Can you work these out from the drawing? Everything is in mm from the part's minimum corner. A direction names the side the tool comes from. Round coordinates to 2 decimals unless told otherwise and drop trailing zeros. Order: outer loops, then holes, each group sorted by start corner. A loop starts at its lowest first (then second) coordinate and runs counter-clockwise, first axis right, second up. Notation, with made-up numbers: M 61.5,-31 L 108.5,-31 A24 cw 108.5,-12 Z; hole C -1,-32.5 d8. An arc over 180 degrees is marked long. Write each question's results on one line, items separated by ' | '. Start each with the question number.
1. Suppose I cut it at C-C on z = 20. Write out the boundary of the cut face in (x, y).
2. We'd pull the mould along Y, two halves only. Please class the marked faces 3, 4, 5 and 6: released by +Y, released by -Y, zero draft, split by the parting line, or undercut.
3. Suppose I cut it at A-A on y = 50. Write out the boundary of the cut face in (x, z).
4. Suppose I cut it at B-B on x = 67.5. Write out the boundary of the cut face in (y, z).
5. I'm going to push flat-ended pins straight in: pin 1 (8 mm diameter, centred on y = 6.5, z = 43.5, fed in from -X); pin 2 (10 mm diameter, centred on y = 52.5, z = 20.5, fed in from +X); pin 3 (9.5 mm diameter, centred on x = 61.5, y = 14, fed in from -Z). Where does each tip first touch, or does it pass through?
6. Please list where these lines run through material, in increasing order: L1, parallel to Y at x = 67, z = 51 (3 decimals); L2, parallel to X at y = 30, z = 43.5; L3, parallel to Y at x = 60.5, z = 12.5.
7. Suppose I cut it at D-D on y = 30. Write out the boundary of the cut face in (x, z).
8. For the marked faces 1 and 2, which set-ups out of +Z, -Z, +X, -X, +Y, -Y let a thin tool reach every point of the face, with its end or its side?
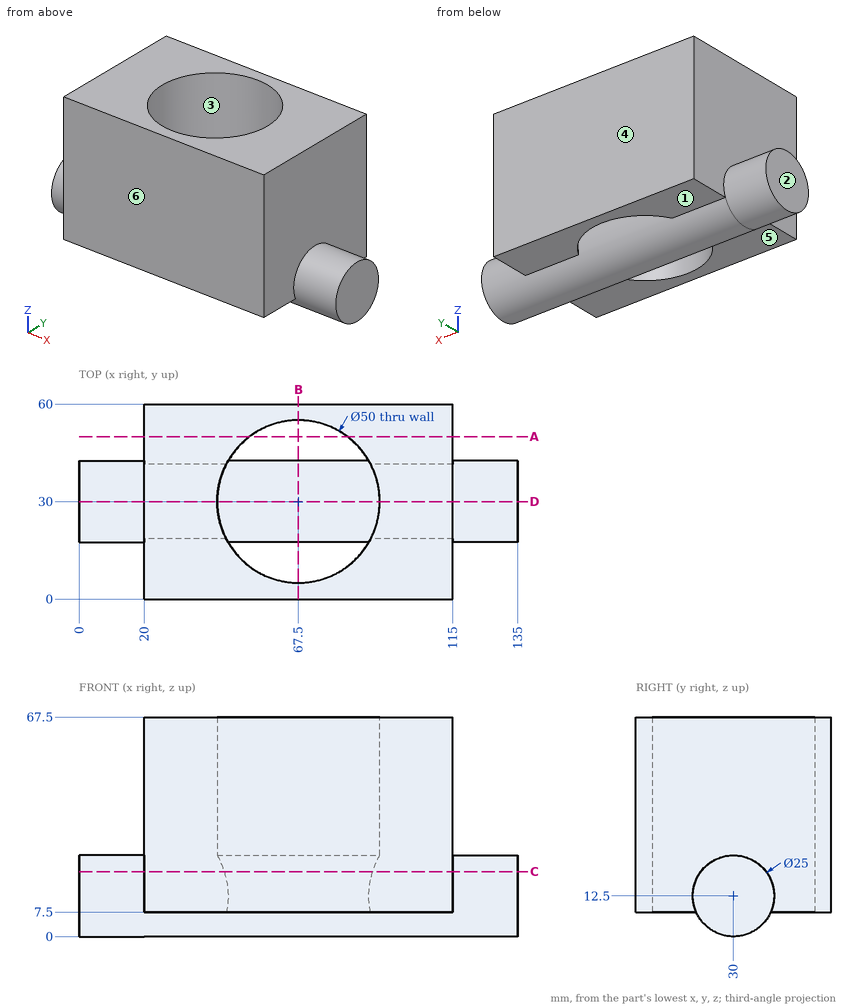
Filled sheet:
1) outline: M 0,20 L 20,20 L 20,0 L 115,0 L 115,20 L 135,20 L 135,40 L 115,40 L 115,60 L 20,60 L 20,40 L 0,40 Z; hole M 44.59,20 A25 ccw 90.41,20 Z; hole M 44.59,40 L 90.41,40 A25 ccw Z
2) face 3: undercut | face 4: released by +Y | face 5: zero draft | face 6: released by -Y
3) outline: M 20,7.5 L 52.5,7.5 L 52.5,67.5 L 20,67.5 Z; M 82.5,7.5 L 115,7.5 L 115,67.5 L 82.5,67.5 Z
4) outline: M 0,7.5 L 5,7.5 L 5,67.5 L 0,67.5 Z; C 30,12.5 d25; M 55,7.5 L 60,7.5 L 60,67.5 L 55,67.5 Z
5) pin 1: stops at x = 20 | pin 2: stops at x = 115 | pin 3: stops at z = 7.05
6) L1: y = 0 to 5.005, 54.995 to 60 | L2: x = 20 to 42.5, 92.5 to 115 | L3: y = 0 to 6, 17.5 to 42.5, 54 to 60
7) outline: M 0,0 L 135,0 L 135,25 L 115,25 L 115,67.5 L 92.5,67.5 L 92.5,25 L 42.5,25 L 42.5,67.5 L 20,67.5 L 20,25 L 0,25 Z
8) face 1: -Z, +X, -X, +Y | face 2: +Z, -Z, -X, +Y, -Y
